Model file for the job. Use its own axes, mm. A direction names the side the tool comes from. Coordinates: 2 decimals unless noted, no trailing zeros. Order: outer loops, then holes, each group sorted by start corner. A loop starts at its lowest first (then second) coordinate and runs counter-clockwise, first axis right, second up. Notation, with made-up numbers: (-15, -28) -> (17, -28) arc R17 ccw to (17, -5) -> close; hole circle Ø6 at (14, 4). An arc over 180 degrees is marked (long way). Use CSV: the item, a comma, the result in double quotes. Start each with the question number.
(1) Cut at C-C on z = -2.25. Write the cut outline in (x, y), plus the area to 3 significant figures.
(2) Tool access for faces 4 (the cylindrical face through (-9.646, -12.13, -9.84)), 5 (the cylindrical face through (-9.8, -2.773, -4.325)): list every direction of +Z, -Z, +X, -X, +Y, -Y with a clear straight run to the whole face (end or side of a thin tool).
(3) Cut at B-B on y = -12. Write the cut outline in (x, z) (3 decimals), plus the area to 3 significant figures.
(4) Pin check, flat tips, straight feed: pin 1 Ø7.5 at (y, z) = (4, -4) entering from -X; pin 2 Ø4 at (x, z) = (-7.5, -7.5) entering from -Y; pin 3 Ø1.9 at (y, z) = (-2.5, -6.5) entering from +X (3 decimals); pin 4 Ø5 at (x, z) = (-7.5, -7.5) entering from +Y. Stop position of each tip, or through.
(5) Cut at D-D on x = -29. Give the number of separate pieces and of enclosed holes in the cut face, plus the area to 3 significant figures.
(6) Probe L1, parallel to Y at x = -29.35, z = -7.5; L2, parallel to Y at x = -3.75, z = -7.5 (3 decimals); L3, parallel to Z at x = -7.5, y = 0.5 (3 decimals). List the from-to ranges inside material, lowest first.
(7) Cut at A-A on x = -13.5. Write the cut outline in (y, z).
(8) Pull direction Z, two halves, no side cores. Call faces 1 (the flat face through (-23, -33, -7)), 2 (the cylindrical face through (-14.77, -20.64, -8.98)), 3 (the cylindrical face through (-29.69, -27.76, -13.09)): pulls with the +Z half, pulls with the -Z half, needs draft (parallel to the pull), parting line crosses it, or undercut.
Autodesk Inventor part; units mm, degrees
ref_plane "YZ Plane" through (0, 0, 0) normal (1, 0, 0) x (0, 1, 0)
ref_plane "XZ Plane" through (0, 0, 0) normal (0, 1, 0) x (-1, 0, 0)
ref_plane "XY Plane" through (0, 0, 0) normal (0, 0, 1) x (1, 0, 0)
sketch "Base Profile" plane through (0, 0, 0) normal (0, 1, 0) x (-1, 0, 0)
  line L0 (0, 0) -> (15, 0)
  line L1 (15, 0) -> (15, -15)
  line L2 (15, -15) -> (0, -15)
  line L3 (0, -15) -> (0, 0)
  line L4 (15, 0) -> (31.5, 0)
  line L5 (31.5, 0) -> (31.5, -15)
  line L6 (31.5, -15) -> (15, -15)
  line L7 (15, -15) -> (15, 0)
  dimension "d164" = 15
  dimension "d165" = 15
  dimension "d166" = 16.5
  dimension "d167" = 15
extrude "Stock" add sketch "Base Profile" against normal blind 33
extrude "Top Extrusion Post" add sketch "Base Profile" along normal blind 15 contours L0 L1 L2 L3
extrude "Lower Extrusion Post" add sketch "Base Profile" against normal blind 22.5 from surface at -33 contours L0 L1 L2 L3
sketch "Sketch27" plane through (0, -33, -15) normal (0, 0, -1) x (-1, 0, 0)
  line L0 (0, -22.5) -> (0, 48)
  line L1 (31.5, 0) -> (15, 0)
  line L2 (31.5, 33) -> (31.5, 0)
  line L3 (15, 33) -> (31.5, 33)
  line L4 (15, 33) -> (15, 48)
  line L5 (0, 48) -> (15, 48)
  line L6 (0, 25.5) -> (31.5, 25.5)
  line L7 (0, 16.5) -> (31.5, 16.5)
  line L8 (15, 33) -> (15, 0)
  line L9 (0, -22.5) -> (15, -22.5)
  line L10 (15, 0) -> (15, -22.5)
  point P0 (15, 25.5)
  point P1 (15, 16.5)
  dimension "d373" = 7.5
  dimension "d374" = 16.5
extrude "Lower Half Cut" cut sketch "Sketch27" against normal through all contours L8 L6 L2 L7
sketch "Bottom Profile" plane through (-35, -33, -15) normal (0, -1, 0) x (1, 0, 0)
  line L0 (13.5, 7.5) -> (10, 7.5) construction
  line L1 (13.5, 10.675) -> (10, 10.675)
  line L2 (10, 4.325) -> (13.5, 4.325)
  arc A0 (13.5, 4.325) -> (13.5, 10.675) centre (13.5, 7.5) ccw
  arc A1 (10, 10.675) -> (10, 4.325) centre (10, 7.5) ccw
  line L3 (3.5, 15) -> (3.5, 0)
  line L4 (35, 15) -> (3.5, 15)
  point P0 (11.75, 7.5)
  dimension "d291" = 3.5
  dimension "d292" = 6.35
  dimension "d293" = 6.5
  dimension "d294" = 7.5
extrude "Slot Cut" cut sketch "Bottom Profile" along normal blind 24 from surface at -33
sketch "Front Hole Pattern" plane through (0, -33, 0) normal (1, 0, 0) x (0, 0, -1)
  line L0 (0, 0) -> (0, 48) construction
  circle A0 centre (7.5, 40.5) radius 3.175
  line L1 (0, 48) -> (15, 48) construction
  circle A1 centre (7.5, 30.25) radius 3.175
  circle A2 centre (7.5, -7.5) radius 3.175
  circle A3 centre (7.5, 11.75) radius 3.175
  line L2 (15, -22.5) -> (15, 48) construction
  line L3 (0, 33) -> (15, 33) construction
  line L4 (0, 25.5) -> (15, 25.5) construction
  line L5 (0, 16.5) -> (15, 16.5) construction
  line L6 (0, 27.5) -> (15, 27.5) construction
  line L7 (0, 14.5) -> (15, 14.5) construction
  line L8 (0, 9) -> (15, 9) construction
  line L9 (15, 0) -> (0, 0) construction
  dimension "d317" = 6.35
  dimension "d318" = 7.5
  dimension "d319" = 7.5
  dimension "d354" = 6.35
  dimension "d369" = 6.35
  dimension "d371" = 6.35
  dimension "d377" = 15
  dimension "d378" = 7.5
  dimension "d379" = 9
  dimension "d380" = 2
  dimension "d381" = 2.75
  dimension "d382" = 2
  dimension "d383" = 7.5
  dimension "d384" = 2.75
  dimension "d385" = 7.5
hole "Front Adjustment Hole" at (0, -2.75, -7.5) at (0, -21.25, -7.5) direction (-1, 0, 0) diameter 3.2004 end through all counterbore diameter 6.35 counterbore depth 10.675
hole "Front Mounting Hole" at (0, 7.5, -7.5) at (0, -40.5, -7.5) direction (-1, 0, 0) diameter 3.2004 end through all counterbore diameter 6.35 counterbore depth 10.675
sketch "Sketch33" plane through (0, 15, 0) normal (0, 1, 0) x (1, 0, 0)
  line L0 (-15, 15) -> (-15, 0)
  line L1 (-15, 0) -> (0, 0)
  line L2 (0, 0) -> (0, 15)
  line L3 (0, 15) -> (-15, 15)
  circle A0 centre (-7.5, 7.5) radius 3.175
  dimension "d340" = 6.35
  dimension "d341" = 7.5
  dimension "d342" = 7.5
hole "Top Mounting Hole" at (-7.5, 15, -7.5) direction (0, -1, 0) diameter 3.2004 end through all counterbore diameter 6.35 counterbore depth 61.674
fillet "Fillet2" radius 6.35 2 edges at (-31.5, -3.75, -15) (-31.5, -24.75, -15)
equation "\"d164\" = extrusionWidth"
equation "\"d165\" = extrusionWidth"
equation "\"d166\" = idlerLength"
equation "\"d167\" = d165"
equation "\"d168\" = extrusionOffset"
equation "\"extrusionWidth\" = 15"
equation "\"idlerLength\" = 16.5"
equation "\"bearingOffsetFromBottom\" = 7.5"
equation "\"extrusionOffset\" = 33"
equation "\"bearingStackHeight\" = 9"
equation "\"bearingSlotLength\" = 3.5"
equation "\"bearingClearance\" = 13"
equation "\"pinSupportLength\" = 2"
properties part number "A Idler" material "Aluminum 6061"
Outcome:
1,outline,"(-31.5, -33) -> (-15, -33) -> (-15, -55.5) -> (0, -55.5) -> (0, 15) -> (-15, 15) -> (-15, 0) -> (-31.5, 0) -> (-31.5, -7.5) -> (-15, -7.5) -> (-15, -16.5) -> (-31.5, -16.5) -> close"
1,area,"1,450 mm2"
2,face 4,"+Y"
2,face 5,"+X"
3,outline,"(-15, -15) -> (0, -15) -> (0, 0) -> (-15, 0) -> close; hole circle Ø6.35 at (-7.5, -7.5)"
3,area,"193 mm2"
4,pin 1,"x = -15"
4,pin 2,"y = -55.5"
4,pin 3,"x = -10.675"
4,pin 4,"y = -46.67"
5,separate pieces,"2"
5,enclosed holes,"2"
5,area,"313 mm2"
6,L1,"-33 to -22.85, -19.65 to -16.5, -7.5 to -4.35, -1.15 to 0"
6,L2,"-55.5 to -43.675, -37.325 to -24.425, -18.075 to -5.925, 0.425 to 4.325, 10.675 to 15"
6,L3,"-15 to -10.675, -4.325 to 0"
7,outline,"(-55.5, -15) -> (15, -15) -> (15, 0) -> (-55.5, 0) -> close; hole circle Ø3.2 at (-40.5, -7.5); hole circle Ø3.2 at (-21.25, -7.5); hole circle Ø3.2 at (-2.75, -7.5); hole circle Ø3.2 at (7.5, -7.5)"
8,face 1,"needs draft"
8,face 2,"undercut"
8,face 3,"pulls with the -Z half"
